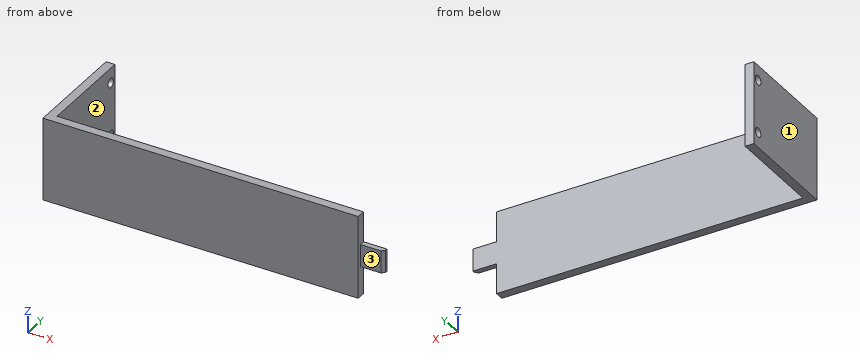
```python
from build123d import *

# Parameters (mm, degrees)
SKETCH1_W           = 107
SKETCH1_H           = 28.15
BOSS_EXTRUDE1_DEPTH = 3
SKETCH2_W           = 7.6
SKETCH2_H           = 1.8
BOSS_EXTRUDE2_DEPTH = 8
CHAMFER1_SIZE       = 1
SKETCH3_W           = 3
SKETCH3_H           = 28.15
BOSS_EXTRUDE3_DEPTH = 33.25
SKETCH4_R           = 1.6
CUT_EXTRUDE1_DEPTH  = 33.25


with BuildPart() as part:
    # Sketch1 → Boss-Extrude1 (new body)
    with BuildSketch(Plane(origin=(0, 0, 0), x_dir=(1, 0, 0), z_dir=(0, 1, 0))):
        with Locations((3.889337641, -2.752705977)):
            Rectangle(SKETCH1_W, SKETCH1_H)
    extrude(amount=BOSS_EXTRUDE1_DEPTH)

    # Sketch2 → Boss-Extrude2 (add)
    with BuildSketch(Plane(origin=(57.389337641, 0, 0), x_dir=(0, 0, -1), z_dir=(1, 0, 0))):
        with Locations((-2.752705977, 2.1)):
            Rectangle(SKETCH2_W, SKETCH2_H)
    extrude(amount=BOSS_EXTRUDE2_DEPTH)

    # Chamfer1
    chamfer1_edges = [part.edges().sort_by_distance(p)[0] for p in [
        (65.389337641, 1.2, 2.752705977),
    ]]
    chamfer(chamfer1_edges, length=CHAMFER1_SIZE)

    # Sketch3 → Boss-Extrude3 (add)
    with BuildSketch(Plane(origin=(0, 3, 0), x_dir=(1, 0, 0), z_dir=(0, 1, 0))):
        with Locations((-48.110662359, -2.752705977)):
            Rectangle(SKETCH3_W, SKETCH3_H)
    extrude(amount=BOSS_EXTRUDE3_DEPTH)

    # Sketch4 → Cut-Extrude1 (cut)
    with BuildSketch(Plane.ZY.offset(49.610662359)):
        with Locations((-6.247294023, 33.85)):
            Circle(SKETCH4_R)
        with Locations((11.752705977, 33.85)):
            Circle(SKETCH4_R)
    extrude(amount=-CUT_EXTRUDE1_DEPTH, mode=Mode.SUBTRACT)


solid = part.part
```
Build history of the part. All positions in model axes, mm. Face numbers are marked on the shaded views. A direction names the side the tool comes from. Round coordinates to 2 decimals unless told otherwise and drop trailing zeros. Write each loop counter-clockwise with the first axis right and the second up, starting at its lowest first coordinate (ties: lowest second). Pieces come first, ordered by that corner, then holes.
1) Pin check, flat tips, straight feed: pin 1 (8.5 mm diameter, centred on y = 23.5, z = -2.5, fed in from +X); pin 2 (14 mm diameter, centred on x = 3, z = 7, fed in from +Y); pin 3 (0.9 mm diameter, centred on x = 61.5, y = 2, fed in from -Z); pin 4 (3 mm diameter, centred on y = 33.85, z = -6.25, fed in from -X). Stop position of each tip, or through.
2) Band-saw the part on C-C, the plane z = 0.5. List the corners of the cut face in (x, y), and give its area (3 significant figures).
3) Band-saw the part on B-B, the plane z = -6.5. List the corners of the cut face in (x, y).
4) Drill centre lines: probe 1 along Z at (x, y) = (-47, 33); probe 2 along X at (y, z) = (16, -7); probe 3 along Y at (x, z) = (-34, 0.5). Where is each one in solid material? Low to high.
5) 3-axis set-ups, long thin cutter, end or side, ignore diameter. For the marked faces 1, 2 and 3: which of +Z, -Z, +X, -X, +Y, -Y reach the whole face in a straight line?
6) Band-saw the part on D-D, the plane x = 22. List the corners of the cut face in (y, z), and give its area (4 significant figures).
7) Band-saw the part on A-A, the plane y = 33.85. List the corners of the cut face in (x, z).
Ans:
1. pin 1: stops at x = -46.61
1. pin 2: stops at y = 3
1. pin 3: stops at z = -1.05
1. pin 4: passes through
2. outline: (-49.61, 0) - (57.39, 0) - (57.39, 1.2) - (64.39, 1.2) - (65.39, 2.2) - (65.39, 3) - (-46.61, 3) - (-46.61, 36.25) - (-49.61, 36.25) - close
2. area: 435 mm2
3. outline: (-49.61, 0) - (57.39, 0) - (57.39, 3) - (-46.61, 3) - (-46.61, 32.27) - (-49.61, 32.27) - close; (-49.61, 35.43) - (-46.61, 35.43) - (-46.61, 36.25) - (-49.61, 36.25) - close
4. probe 1: z = -11.32 to -7.6, -4.89 to 10.4, 13.11 to 16.83
4. probe 2: x = -49.61 to -46.61
4. probe 3: y = 0 to 3
5. face 1: +Z, -Z, -X, +Y, -Y
5. face 2: +Z, -Z, +X, +Y
5. face 3: +Z, -Z, +X, -Y
6. outline: (0, -11.32) - (3, -11.32) - (3, 16.83) - (0, 16.83) - close
6. area: 84.45 mm2
7. outline: (-49.61, -11.32) - (-46.61, -11.32) - (-46.61, -7.85) - (-49.61, -7.85) - close; (-49.61, -4.65) - (-46.61, -4.65) - (-46.61, 10.15) - (-49.61, 10.15) - close; (-49.61, 13.35) - (-46.61, 13.35) - (-46.61, 16.83) - (-49.61, 16.83) - close
